```python
from build123d import *

# Parameters (mm, degrees)
SKETCH1_R               = 20.32
BOSS_EXTRUDE1_DEPTH     = 50.8
SHELL1_T                = -3.175
SKETCH2_R               = 4.064
CUT_EXTRUDE1_DEPTH      = 56.623245366
CUT_EXTRUDE1_DEPTH_BACK = 46.482


with BuildPart() as part:
    # Sketch1 → Boss-Extrude1 (new body)
    with BuildSketch(Plane(origin=(0, 0, 0), x_dir=(1, 0, 0), z_dir=(0, 1, 0))):
        with Locations(Location((0, 0, 0), (0, 0, 270))):
            Circle(SKETCH1_R)
    extrude(amount=BOSS_EXTRUDE1_DEPTH)

    # Shell1
    shell1_openings = [part.faces().sort_by_distance(p)[0] for p in [
        (0, 50.8, 0),
    ]]
    offset(amount=SHELL1_T, openings=shell1_openings, kind=Kind.INTERSECTION)

    # Sketch2 → Cut-Extrude1 (cut, two sides)
    with BuildSketch(Plane(origin=(0, 3.175, 0), x_dir=(1, 0, 0), z_dir=(0, 1, 0))) as cut_extrude1_sk:
        with Locations(Location((0, 0, 0), (0, 0, 270))):
            Circle(SKETCH2_R)
    extrude(amount=CUT_EXTRUDE1_DEPTH, mode=Mode.SUBTRACT)
    extrude(cut_extrude1_sk.sketch, amount=-CUT_EXTRUDE1_DEPTH_BACK, mode=Mode.SUBTRACT)


solid = part.part
```
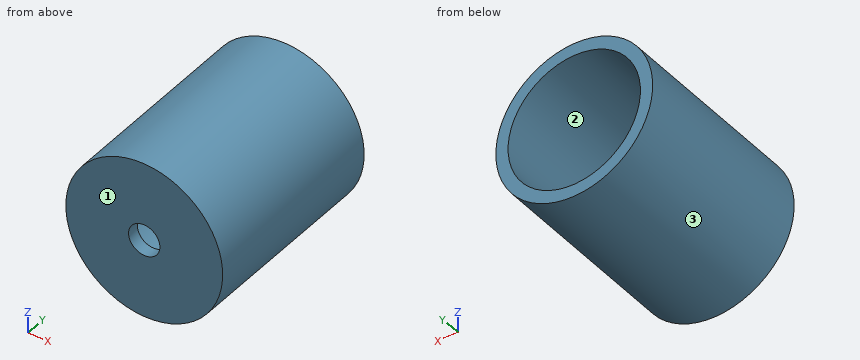
For this review, take the finished solid that the model builds, in its own axes (mm). Face numbers are marked on the shaded views. Coordinates: 2 decimals unless noted, no trailing zeros. Loops run counter-clockwise (first coordinate to the right, second up) from the corner with the lowest first, then second, coordinate; pieces in that order, holes last.
1. Add section B-B, the plane z = 0. Give the boundary of the cut face in (x, y) (3 decimals), then the cut area to 3 significant figures.
2. Insertion check: P1, Ø1.5, axis at y = 15.5, z = -5.5, coming from the +X side; P2, Ø12, axis at x = -15.5, y = 18, coming from the -Z side; P3, Ø8, axis at x = -8.5, z = 12.5, coming from the -Y side; P4, Ø4, axis at y = 16, z = 2, coming from the +X side. Each pin has a flat end and moves straight along its axis. Give the tip position at first contact, or say it passes through.
3. For line 1 (X direction, y = 31, z = 0) (3 decimals); line 2 (X direction, y = 1, z = 0); line 3 (Z direction, x = 7, y = 8.5), list the stretches that pass through material, from the lowest coordinate up.
4. Add section D-D, the plane y = 28. Give the boundary of the cut face in (x, z) (3 decimals).
5. Add section A-A, the plane x = 0. Give the boundary of the cut face in (y, z) (3 decimals), then the cut area to 3 significant figures.
6. Add section C-C, the plane z = 10. Give the boundary of the cut face in (x, y) (3 decimals).
7. Mouldability with a two-part tool opening along X and no side actions: class the marked faces 1, 2 and 3 as +X half, -X half, draft (parallel to the pull), parting line (faces both ways), or undercut.
Result:
1. outline: (-20.32, 0) - (-4.064, 0) - (-4.064, 3.175) - (-17.145, 3.175) - (-17.145, 50.8) - (-20.32, 50.8) - close; (4.064, 0) - (20.32, 0) - (20.32, 50.8) - (17.145, 50.8) - (17.145, 3.175) - (4.064, 3.175) - close
1. area: 406 mm2
2. P1: stops at x = 19.76
2. P2: stops at z = -17.96
2. P3: stops at y = 0
2. P4: stops at x = 20.32
3. line 1: x = -20.32 to -17.145, 17.145 to 20.32
3. line 2: x = -20.32 to -4.06, 4.06 to 20.32
3. line 3: z = -19.08 to -15.65, 15.65 to 19.08
4. outline: circle Ø40.64 at (0, 0); hole circle Ø34.29 at (0, 0)
5. outline: (0, -20.32) - (50.8, -20.32) - (50.8, -17.145) - (3.175, -17.145) - (3.175, -4.064) - (0, -4.064) - close; (0, 4.064) - (3.175, 4.064) - (3.175, 17.145) - (50.8, 17.145) - (50.8, 20.32) - (0, 20.32) - close
5. area: 406 mm2
6. outline: (-17.689, 0) - (17.689, 0) - (17.689, 50.8) - (13.927, 50.8) - (13.927, 3.175) - (-13.927, 3.175) - (-13.927, 50.8) - (-17.689, 50.8) - close
7. face 1: draft
7. face 2: undercut
7. face 3: parting line
